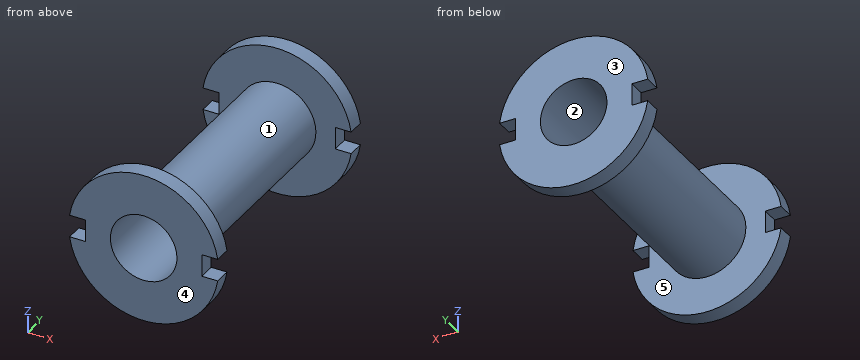
```python
from build123d import *

# Parameters (mm, degrees)
SKETCH_1_R          = 6.75
SKETCH_1_R_2        = 3
EXTRUDE_1_DEPTH     = 11.5
SKETCH_2_R          = 11.31533916
SKETCH_2_R_2        = 3.5
CUT_EXTRUDE_1_DEPTH = 10
SKETCH_4_W          = 3
SKETCH_4_H          = 2
CUT_EXTRUDE_2_DEPTH = 25.90230913


with BuildPart() as part:
    # 草图1 → 凸台-拉伸1 (new, symmetric)
    with BuildSketch(Plane(origin=(0, 0, 0), x_dir=(1, 0, 0), z_dir=(0, 1, 0))):
        with Locations(Location((0, 0, 0), (0, 0, 270))):
            Circle(SKETCH_1_R)
        with Locations(Location((0, 0, 0), (0, 0, 270))):
            Circle(SKETCH_1_R_2, mode=Mode.SUBTRACT)
    extrude(amount=EXTRUDE_1_DEPTH, both=True)

    # 草图2 → 切除-拉伸1 (cut, symmetric)
    with BuildSketch(Plane(origin=(0, 0, 0), x_dir=(1, 0, 0), z_dir=(0, 1, 0))):
        Circle(SKETCH_2_R)
        with Locations(Location((0, 0, 0), (0, 0, 270))):
            Circle(SKETCH_2_R_2, mode=Mode.SUBTRACT)
    extrude(amount=CUT_EXTRUDE_1_DEPTH, both=True, mode=Mode.SUBTRACT)

    # 草图4 → 切除-拉伸2 (cut, through all)
    with BuildSketch(Plane(origin=(0, 11.5, 0), x_dir=(1, 0, 0), z_dir=(0, 1, 0))):
        with Locations((-6.75, 0)):
            Rectangle(SKETCH_4_W, SKETCH_4_H)
        with Locations((6.75, 0)):
            Rectangle(SKETCH_4_W, SKETCH_4_H)
    extrude(amount=-CUT_EXTRUDE_2_DEPTH, mode=Mode.SUBTRACT)


solid = part.part
```
The listing builds one solid part. Answer for the finished solid, in the listing's coordinates (mm). Face numbers are marked on the shaded views. A direction names the side the tool comes from. Round coordinates to 2 decimals unless told otherwise and drop trailing zeros. Order: outer loops, then holes, each group sorted by start corner. A loop starts at its lowest first (then second) coordinate and runs counter-clockwise, first axis right, second up. Notation, with made-up numbers: (5.5, 12.5) - (22.5, 12.5) arc R28 cw to (22.5, 33.5) - close; hole circle Ø2 at (24, -8). An arc over 180 degrees is marked (long way). Put each result on its own line as item: value. Start each with the question number.
(1) Straight lines are drawn through the part: probe 1 along X at (y, z) = (5.25, 0); probe 2 along Y at (x, z) = (-2.75, 5); probe 3 along Z at (x, y) = (-2.25, -3.5). For each, find the intervals that lie inside material, in ascending order. Write a range as from..to.
(2) Find section A-A (x = 0). Give the vertices of the cut face in (y, z).
(3) For the marked faces 1 and 2, determine the directions among +Z, -Z, +X, -X, +Y, -Y from which every point of the face is accessible in a straight line to the end or side of a thin tool.
(4) Determine the mould class of the marked faces 3, 4 and 5 for opening direction Y: released by +Y, released by -Y, zero draft, split by the parting line, or undercut.
(5) Find section B-B (z = 0). Give the vertices of the cut face in (x, y), plus the area to 3 significant figures.
(6) Given P1, Ø1.6, axis at x = 6.5, y = -10.5, coming from the -Z side; P2, Ø1.6, axis at x = 6, y = -10.5, coming from the +Z side; P3, Ø3, axis at y = 1, z = 1.5, coming from the -X side, each flat-ended and moving along its own axis, determine where each tip first touches the part or whether it passes through.
(7) Find section C-C (y = -2). Give the vertices of the cut face in (x, z).
(8) Find section D-D (z = -4.75). Give the vertices of the cut face in (x, y).
Reply:
1. probe 1: -3.5..-3, 3..3.5
1. probe 2: -11.5..-10, 10..11.5
1. probe 3: -2.68..-1.98, 1.98..2.68
2. outline: (-11.5, -6.75) - (-10, -6.75) - (-10, -3.5) - (10, -3.5) - (10, -6.75) - (11.5, -6.75) - (11.5, -3) - (-11.5, -3) - close; (-11.5, 3) - (11.5, 3) - (11.5, 6.75) - (10, 6.75) - (10, 3.5) - (-10, 3.5) - (-10, 6.75) - (-11.5, 6.75) - close
3. face 1: none
3. face 2: +Y, -Y
4. face 3: released by +Y
4. face 4: released by -Y
4. face 5: undercut
5. outline: (-5.25, -11.5) - (-3, -11.5) - (-3, 11.5) - (-5.25, 11.5) - (-5.25, 10) - (-3.5, 10) - (-3.5, -10) - (-5.25, -10) - close; (3, -11.5) - (5.25, -11.5) - (5.25, -10) - (3.5, -10) - (3.5, 10) - (5.25, 10) - (5.25, 11.5) - (3, 11.5) - close
5. area: 33.5 mm^2
6. P1: z = -3.62
6. P2: z = 4.3
6. P3: x = -3.5
7. outline: circle Ø7 at (0, 0); hole circle Ø6 at (0, 0)
8. outline: (-4.8, -11.5) - (4.8, -11.5) - (4.8, -10) - (-4.8, -10) - close; (-4.8, 10) - (4.8, 10) - (4.8, 11.5) - (-4.8, 11.5) - close
